Read the model definition and answer for the solid it produces. Units are mm, in the model's axes. A direction names the side the tool comes from. Give positions to 0.01 mm unless a question says otherwise; leave off trailing zeros. Write each loop counter-clockwise with the first axis right and the second up, starting at its lowest first coordinate (ties: lowest second). Pieces come first, ordered by that corner, then holes. Notation, with made-up numbers: (67, 16) -> (73, 16) arc R26 ccw to (73, 35) -> close; hole circle Ø2 at (46, -32). An arc over 180 degrees is marked (long way). Put each result on its own line as item: value. Start each with the question number.
from build123d import *

# Parameters (mm, degrees)
SKETCH_2_R               = 1.5
CUT_EXTRUDE_1_DEPTH      = 3
SKETCH_3_W               = 0.5
SKETCH_3_H               = 3
EXTRUDE_1_DEPTH          = 2
EXTRUDE_START            = 1.5
SKETCH_4_R               = 12.5
EXTRUDE_2_DEPTH          = 1.5
SKETCH_5_R               = 0.5
EXTRUDE_3_DEPTH          = 1
SKETCH_6_R               = 7
EXTRUDE_4_DEPTH          = 5
SKETCH_7_W               = 5
SKETCH_7_H               = 9.498376428
EXTRUDE_5_DEPTH          = 3
CHAMFER_1_SIZE           = 0.2
CUT_EXTRUDE_2_DEPTH      = 38.251363929
CUT_EXTRUDE_2_DEPTH_BACK = 38.251363929
SKETCH_8_W               = 7
SKETCH_8_H               = 0.45


with BuildPart() as part:
    # 草图1 → 旋转1 (revolve)
    with BuildSketch(Plane.XY, mode=Mode.PRIVATE) as revolve_1_sk:
        Polygon((0, 12), (0, 12.5), (-19.5, 12.5), (-19.5, 0), (19.5, 0), (32.5, 0), (32.5, 1.5), (21.5, 1.5), (21.5, 3.5), (19.5, 3.5), (19.5, 12), align=None)
    revolve(revolve_1_sk.sketch.rotate(Axis((-61.965581957, 0, 0), (1, 0, 0)), 90), axis=Axis((-61.965581957, 0, 0), (1, 0, 0)))

    # 草图2 → 切除-拉伸1 (cut)
    with BuildSketch(Plane(origin=(19.5, 0, 0), x_dir=(0, 0, -1), z_dir=(1, 0, 0))):
        with Locations((0, -8.5)):
            Circle(SKETCH_2_R)
        with Locations(Location((0, 8.5, 0), (0, 0, 180))):
            Circle(SKETCH_2_R)
    extrude(amount=-CUT_EXTRUDE_1_DEPTH, mode=Mode.SUBTRACT)

    # 草图3 → 凸台-拉伸1 (add)
    with BuildSketch(Plane.ZY.offset(19.5)):
        with Locations((-9.404663304, 0)):
            Rectangle(SKETCH_3_W, SKETCH_3_H)
        with Locations((9.404663304, 0)):
            Rectangle(SKETCH_3_W, SKETCH_3_H)
    extrude(amount=EXTRUDE_1_DEPTH)

    # 草图4 → 凸台-拉伸2 (add)
    with BuildSketch(Plane.ZY.offset(21.5).offset(EXTRUDE_START)):
        Circle(SKETCH_4_R)
    extrude(amount=-EXTRUDE_2_DEPTH)

    # 草图5 → 凸台-拉伸3 (add)
    with BuildSketch(Plane.ZY.offset(23)):
        Circle(SKETCH_5_R)
    extrude(amount=EXTRUDE_3_DEPTH)

    # 草图6 → 凸台-拉伸4 (add)
    with BuildSketch(Plane.ZY.offset(24)):
        Circle(SKETCH_6_R)
    extrude(amount=EXTRUDE_4_DEPTH)

    # 草图7 → 凸台-拉伸5 (add)
    with BuildSketch(Plane.ZY.offset(23)):
        with Locations((-10.734958049, 0)):
            Rectangle(SKETCH_7_W, SKETCH_7_H)
    extrude(amount=EXTRUDE_5_DEPTH)

    # 倒角1
    chamfer_1_edges = [part.edges().sort_by_distance(p)[0] for p in [
        (-29, 0, -7),
    ]]
    chamfer(chamfer_1_edges, length=CHAMFER_1_SIZE)

    # 草图8 → 切除-拉伸2 (cut, two sides: drawn at the far end of the back side and taken through both)
    with BuildSketch(Plane(origin=(0, 0, 0), x_dir=(1, 0, 0), z_dir=(0, 1, 0)).offset(-CUT_EXTRUDE_2_DEPTH_BACK)):
        with Locations((29, -1.275)):
            Rectangle(SKETCH_8_W, SKETCH_8_H)
    extrude(amount=CUT_EXTRUDE_2_DEPTH + CUT_EXTRUDE_2_DEPTH_BACK, mode=Mode.SUBTRACT)


solid = part.part
1) For faces 4 (the face through (-23, 0, -13)), 5 (the face through (29, 0, 1.05)), 6 (the face through (18, -10, 0)), determine the directions among +Z, -Z, +X, -X, +Y, -Y from which every point of the face is accessible in a straight line to the end or side of a thin tool.
2) For a pull along X with two mould halves and no side action, classify faces 1 (the face through (16.5, 8, 0)), 2 (the face through (-21.5, 0, 0)), 3 (the face through (-26.366, -2.681, 6.466)) as pulls with the +X half, pulls with the -X half, needs draft (parallel to the pull), parting line crosses it, or undercut.
3) Straight lines are drawn through the part: line 1 (Y direction, x = 17.2, z = 0); line 2 (X direction, y = -2, z = -5.75); line 3 (X direction, y = -10.75, z = 1.5). For each, find the intervals that lie inside material, in ascending order. Write a range as [from, to].
4) A cutting plane is placed at A-A on y = 10.75. Give the vertices of the cut face in (x, z).
5) A cutting plane is placed at D-D on x = -1. Give the vertices of the cut face in (y, z).
6) A cutting plane is placed at C-C on y = -8.5. Give the vertices of the cut face in (x, z).
7) Each of these flat-tipped pins is pushed along its axis until it touches: pin 1 Ø5 at (x, z) = (-20.5, 9) entering from -Y; pin 2 Ø1.5 at (x, y) = (-24, 2) entering from +Z; pin 3 Ø5 at (y, z) = (8.5, 0) entering from +X. Where does it stop, or does it pass through?
8) A cutting plane is placed at B-B on x = 15. Give the vertices of the cut face in (y, z).
Results found:
1. face 4: -Z, +X
1. face 5: +Z, +X, +Y, -Y
1. face 6: +X
2. face 1: pulls with the +X half
2. face 2: undercut
2. face 3: needs draft
3. line 1: y = [-12, -10], [-7, 7], [10, 12]
3. line 2: x = [-29, -24], [-23, -21.5], [-19.5, 19.5]
3. line 3: x = [-23, -21.5], [-19.5, 19.5]
4. outline: (-23, -6.38) -> (-21.5, -6.38) -> (-21.5, 6.38) -> (-23, 6.38) -> close; (-19.5, -6.38) -> (0, -6.38) -> (0, -5.33) -> (19.5, -5.33) -> (19.5, 5.33) -> (0, 5.33) -> (0, 6.38) -> (-19.5, 6.38) -> close
5. outline: circle Ø25 at (0, 0)
6. outline: (-23, -9.17) -> (-21.5, -9.17) -> (-21.5, 9.17) -> (-23, 9.17) -> close; (-19.5, -9.17) -> (0, -9.17) -> (0, -8.47) -> (19.5, -8.47) -> (19.5, -1.5) -> (16.5, -1.5) -> (16.5, 1.5) -> (19.5, 1.5) -> (19.5, 8.47) -> (0, 8.47) -> (0, 9.17) -> (-19.5, 9.17) -> close
7. pin 1: stops at y = -10.55
7. pin 2: stops at z = 6.89
7. pin 3: stops at x = 19.5
8. outline: circle Ø24 at (0, 0)
